Source: CAD feature listing. Evaluate the final solid. Frame: model axes, mm. A direction names the side the tool comes from. Round coordinates to 2 decimals unless told otherwise and drop trailing zeros. Order: outer loops, then holes, each group sorted by start corner. A loop starts at its lowest first (then second) coordinate and runs counter-clockwise, first axis right, second up. Notation, with made-up numbers: (25.5, 12.5) -> (72.5, 12.5) arc R15 ccw to (72.5, 23.5) -> close; hole circle Ø7 at (-8, 6.25). An arc over 180 degrees is marked (long way). One line per item, written item: value. Start each with the question number.
1) Ray query, L1, parallel to Y at x = 11.5, z = 15.5; L2, parallel to X at y = -12.5, z = 13.5; L3, parallel to X at y = 8, z = 19.75. Return the intervals inside material, ascending.
2) Reachability of faces 4 (the face through (-9.98, 9.34, 15.66)), 5 (the face through (-6.05, -2.43, 20.28)), 6 (the face through (-1, 0, 11.221)) from +Z, -Z, +X, -X, +Y, -Y: full face, straight path, thin tool, end or side. Return the list, or none.
3) Pin query (flat end, axial travel): P1, Ø8, axis at x = -17.5, z = 21.5, coming from the -Y side; P2, Ø4, axis at y = -9, z = 16.5, coming from the -X side; P3, Ø2, axis at x = -11.5, z = 15, coming from the +Y side; P4, Ø3, axis at y = -0.5, z = 17.5, coming from the -X side. Return the tip coordinate at first contact, or that it passes through.
4) Section C-C (z = 24.5). Return the cut outline in (x, y) (3 decimals).
5) Mould query, pull axis Y, two halves, no side actions, for faces 1 (the face through (-1.695, 0.242, 23.179)), 2 (the face through (15.621, 25.164, 15.7)), 3 (the face through (-6.89, 0.25, 20.221)). Classes: pulls with the +Y half, pulls with the -Y half, needs draft (parallel to the pull), parting line crosses it, or undercut.
6) Section A-A (z = 15.5). Return the cut outline in (x, y), and give its area (3 significant figures).
7) Section B-B (x = 8). State how many separate pieces and enclosed holes the cut face has, and give its area (3 significant figures).
```python
from build123d import *

# Parameters (mm, degrees)
SKETCH1_R           = 100
BOSS_EXTRUDE1_DEPTH = 30
FILLET2_R           = 10
SKETCH2_R           = 20
SKETCH2_R_2         = 4.15
BOSS_EXTRUDE2_DEPTH = 50
SCALE1_SCALE        = 0.05
SCALE2_SCALE        = 6


with BuildPart() as part:
    # Sketch1 → Boss-Extrude1 (new body)
    with BuildSketch(Plane.XY):
        Circle(SKETCH1_R)
        with BuildLine():
            Line((-10.606601718, -10.606601718), (-49.497474683, -49.497474683))
            ThreePointArc((-49.497474683, -49.497474683), (-69.64553071, -7.03562734), (-58.396917549, 38.597927675))
            Line((-58.396917549, 38.597927675), (-10.606601718, -10.606601718))
        make_face(mode=Mode.SUBTRACT)
        with BuildLine():
            ThreePointArc((10.606601718, -10.606601718), (13.858192988, -5.740251485), (15, 0))
            Line((15, 0), (70, 0))
            ThreePointArc((70, 0), (33.601511791, -61.407966954), (-37.741097297, -58.954300732))
            Line((-37.741097297, -58.954300732), (10.606601718, -10.606601718))
        make_face(mode=Mode.SUBTRACT)
        with BuildLine():
            ThreePointArc((0, 15), (-5.740251485, 13.858192988), (-10.606601718, 10.606601718))
            Line((-10.606601718, 10.606601718), (-49.497474683, 49.497474683))
            ThreePointArc((-49.497474683, 49.497474683), (20.152118643, 67.036498374), (68.585712798, 14))
            Line((68.585712798, 14), (0, 15))
        make_face(mode=Mode.SUBTRACT)
    extrude(amount=BOSS_EXTRUDE1_DEPTH)

    # Fillet2
    fillet2_edges = [part.edges().sort_by_distance(p)[0] for p in [
        (-100, 0, 0),
        (-100, 0, 30),
    ]]
    fillet(fillet2_edges, radius=FILLET2_R)

    # Sketch2 → Boss-Extrude2 (add)
    with BuildSketch(Plane(origin=(0, 0, 0), x_dir=(-1, 0, 0), z_dir=(0, 0, -1))):
        Circle(SKETCH2_R)
        Circle(SKETCH2_R_2, mode=Mode.SUBTRACT)
    extrude(amount=-BOSS_EXTRUDE2_DEPTH)


with BuildPart() as part_1:
    # Scale1: scaled about (-0.724367868, -0.188947022, 16.030178363)
    add(part.part.scale(SCALE1_SCALE).moved(Location((-0.688149475, -0.179499671, 15.228669445))))


with BuildPart() as part_2:
    # Scale2: scaled about (-0.724367868, -0.188947022, 16.030178363)
    add(part_1.part.scale(SCALE2_SCALE).moved(Location((3.62183934, 0.94473511, -80.150891815))))


solid = part_2.part
```
Findings:
1. L1: -27.62 to -17.36, -0.13 to 4.19, 17.1 to 27.36
1. L2: -27.74 to -17.48, -12.87 to -6.51, 16.46 to 26.73
1. L3: -27.94 to -19.87, -14.68 to -8.64, 18.85 to 26.93
2. face 4: +Z, -Z
2. face 5: +Z
2. face 6: -Z, +X, -X, +Y, -Y
3. P1: y = -26.16
3. P2: x = -29.71
3. P3: y = 28.15
3. P4: x = -30.51
4. outline: circle Ø12 at (-0.507, -0.132); hole circle Ø2.49 at (-0.507, -0.132)
5. face 1: undercut
5. face 2: parting line crosses it
5. face 3: needs draft
6. outline: circle Ø60 at (-0.51, -0.13); hole (-18.03, 11.45) arc R21 ccw to (-15.36, -14.98) -> (-4.75, -4.37) arc R6 cw to (-6.5, -0.42) -> close; hole (-15.36, 14.72) -> (-4.75, 4.11) arc R6 cw to (3.53, 4.31) -> (20.07, 4.07) arc R21 ccw to start; hole (-11.83, -17.82) arc R21 ccw to (20.49, -0.13) -> (5.49, -0.13) arc R6 cw to (-0.13, -6.12) -> close
6. area: 1,760 mm2
7. separate pieces: 3
7. enclosed holes: 0
7. area: 204 mm2
